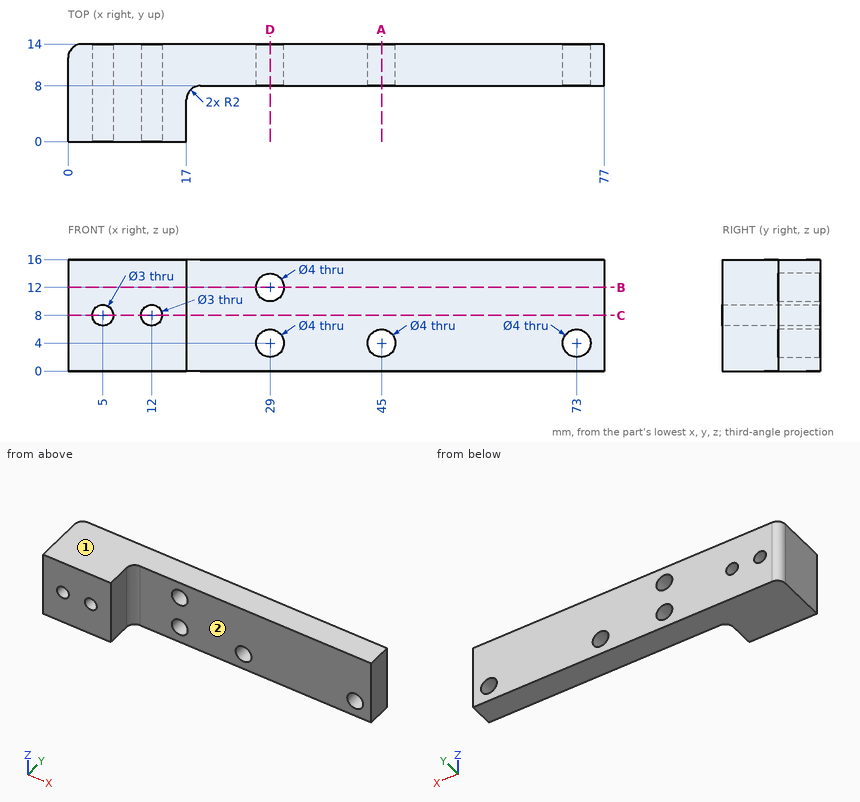
Here's the drawing with two shaded views (mm, measured from the low corner). I have some questions. A direction names the side the tool comes from. Coordinates: 2 decimals unless noted, no trailing zeros. Order: outer loops, then holes, each group sorted by start corner. A loop starts at its lowest first (then second) coordinate and runs counter-clockwise, first axis right, second up.
Item 1: If we section it at D-D on x = 29: List the corners of the cut face in (y, z) for me, plus the area to 3 significant figures.
Result sheet:
outline: (8, 0) - (14, 0) - (14, 2) - (8, 2) - close; (8, 6) - (14, 6) - (14, 10) - (8, 10) - close; (8, 14) - (14, 14) - (14, 16) - (8, 16) - close
area: 48.0 mm2
Item 2: For the marked faces 1 and 2, which set-ups out of +Z, -Z, +X, -X, +Y, -Y let a thin tool reach every point of the face, with its end or its side?
Result sheet:
face 1: +Z, +X, -X, +Y, -Y
face 2: +Z, -Z, +X, -Y
Item 3: For P1, Ø4, axis at x = 23.5, z = 2.5, coming from the -Y side; P2, Ø2.5, axis at x = 5, z = 8, coming from the -Y side; P3, Ø6.5, axis at y = 2.5, z = 9.5, coming from the +X side, each with a flat end and sliding along its axis, tell me the tip position at first contact or that it passes through.
Result sheet:
P1: stops at y = 8
P2: passes through
P3: stops at x = 17
Item 4: If we section it at B-B on z = 12: List the corners of the cut face in (x, y) for me, plus the area to 3 significant figures.
Result sheet:
outline: (0, 0) - (17, 0) - (17, 6) arc R2 cw to (19, 8) - (27, 8) - (27, 14) - (2, 14) arc R2 ccw to (0, 12) - close; (31, 8) - (77, 8) - (77, 14) - (31, 14) - close
area: 574 mm2
Item 5: I need wall thicknesses on line 1 (X direction, y = 10.75, z = 8); line 2 (X direction, y = 4.5, z = 8); line 3 (X direction, y = 9.45, z = 4). Which ranges of each line are inside material? Lowest first, please.
Result sheet:
line 1: x = 0 to 3.5, 6.5 to 10.5, 13.5 to 77
line 2: x = 0 to 3.5, 6.5 to 10.5, 13.5 to 17
line 3: x = 0 to 27, 31 to 43, 47 to 71, 75 to 77
Item 6: If we section it at A-A on x = 45: List the corners of the cut face in (y, z) for me.
Result sheet:
outline: (8, 0) - (14, 0) - (14, 2) - (8, 2) - close; (8, 6) - (14, 6) - (14, 16) - (8, 16) - close
Item 7: If we section it at C-C on z = 8: List the corners of the cut face in (x, y) for me.
Result sheet:
outline: (0, 0) - (3.5, 0) - (3.5, 14) - (2, 14) arc R2 ccw to (0, 12) - close; (6.5, 0) - (10.5, 0) - (10.5, 14) - (6.5, 14) - close; (13.5, 0) - (17, 0) - (17, 6) arc R2 cw to (19, 8) - (77, 8) - (77, 14) - (13.5, 14) - close
